Autodesk Inventor part; units mm, degrees
ref_plane "YZ Plane" through (0, 0, 0) normal (1, 0, 0) x (0, 1, 0)
ref_plane "XZ Plane" through (0, 0, 0) normal (0, 1, 0) x (-1, 0, 0)
ref_plane "XY Plane" through (0, 0, 0) normal (0, 0, 1) x (1, 0, 0)
sketch "Esboço1" plane through (0, 0, 0) normal (0, 1, 0) x (-1, 0, 0)
  line L0 (0, 0) -> (77, 0)
  line L1 (77, 0) -> (77, -140)
  line L2 (77, -140) -> (0, -140)
  line L3 (0, -140) -> (0, 0)
  circle A0 centre (67, -20) radius 2
  circle A1 centre (67, -120) radius 2
  circle A2 centre (26, -20) radius 2
  circle A3 centre (26, -120) radius 2
  dimension "d0" = 77
  dimension "d1" = 140
  dimension "d2" = 4
  dimension "d3" = 4
  dimension "d4" = 4
  dimension "d5" = 4
  dimension "d6" = 10
  dimension "d7" = 10
  dimension "d8" = 20
  dimension "d9" = 20
  dimension "d10" = 20
  dimension "d11" = 20
  dimension "d12" = 26
  dimension "d13" = 26
extrude "Extrusão1" add sketch "Esboço1" along normal blind 8
sketch "Esboço2" plane through (0, 8, 0) normal (0, 1, 0) x (1, 0, 0)
  circle A0 centre (-67, 20) radius 2
  circle A1 centre (-26, 20) radius 2
  circle A2 centre (-26, 120) radius 2
  circle A3 centre (-67, 120) radius 2
  circle A4 centre (-67, 20) radius 4
  circle A5 centre (-67, 120) radius 2
  circle A6 centre (-67, 120) radius 4.5
  circle A7 centre (-26, 120) radius 2
  circle A8 centre (-26, 120) radius 4.5
  circle A9 centre (-26, 20) radius 2
  circle A10 centre (-26, 20) radius 4.5
  point P0 (0, 0)
  dimension "d16" = 8
  dimension "d17" = 9
  dimension "d18" = 9
  dimension "d19" = 9
extrude "Extrusão2" cut sketch "Esboço2" against normal blind 3 contours A3 | A4 | A6 | A8 | A10
sketch "Esboço3" plane through (0, 8, 0) normal (0, 1, 0) x (1, 0, 0)
  point P0 (0, 0)
sketch "Esboço4" plane through (0, 8, 0) normal (0, 1, 0) x (1, 0, 0)
  circle A0 centre (-57, 30) radius 2
  circle A1 centre (-57, 110) radius 2
  circle A2 centre (-67, 20) radius 2
  circle A3 centre (-67, 120) radius 2
  circle A4 centre (-16, 30) radius 2
  circle A5 centre (-16, 110) radius 2
  circle A6 centre (-26, 20) radius 2
  circle A7 centre (-26, 120) radius 2
  point P0 (0, 0)
  dimension "d22" = 4
  dimension "d23" = 4
  dimension "d24" = 10
  dimension "d25" = 10
  dimension "d26" = 10
  dimension "d27" = 10
  dimension "d28" = 4
  dimension "d29" = 4
  dimension "d30" = 10
  dimension "d31" = 10
  dimension "d32" = 10
  dimension "d33" = 10
extrude "Extrusão3" cut sketch "Esboço4" against normal blind 12 contours A0 | A1 | A4 | A5
sketch "Esboço5" plane through (0, 0, 0) normal (0, -1, 0) x (1, 0, 0)
  circle A0 centre (-57, -110) radius 2
  circle A1 centre (-16, -110) radius 2
  circle A2 centre (-16, -30) radius 2
  circle A3 centre (-57, -30) radius 2
  line L0 (-53.525, -112.0063) -> (-57, -114.0126)
  line L1 (-57, -114.0126) -> (-60.475, -112.0063)
  line L2 (-60.475, -112.0063) -> (-60.475, -107.9937)
  line L3 (-60.475, -107.9937) -> (-57, -105.9874)
  line L4 (-57, -105.9874) -> (-53.525, -107.9937)
  line L5 (-53.525, -107.9937) -> (-53.525, -112.0063)
  line L6 (-53.525, -32.0063) -> (-57, -34.0126)
  line L7 (-57, -34.0126) -> (-60.475, -32.0063)
  line L8 (-60.475, -32.0063) -> (-60.475, -27.9937)
  line L9 (-60.475, -27.9937) -> (-57, -25.9874)
  line L10 (-57, -25.9874) -> (-53.525, -27.9937)
  line L11 (-53.525, -27.9937) -> (-53.525, -32.0063)
  line L12 (-16, -105.9874) -> (-12.525, -107.9937)
  line L13 (-12.525, -107.9937) -> (-12.525, -112.0063)
  line L14 (-12.525, -112.0063) -> (-16, -114.0126)
  line L15 (-16, -114.0126) -> (-19.475, -112.0063)
  line L16 (-19.475, -112.0063) -> (-19.475, -107.9937)
  line L17 (-19.475, -107.9937) -> (-16, -105.9874)
  circle A4 centre (-16, -30) radius 2
  line L18 (-12.525, -32.0063) -> (-16, -34.0126)
  line L19 (-16, -34.0126) -> (-19.475, -32.0063)
  line L20 (-19.475, -32.0063) -> (-19.475, -27.9937)
  line L21 (-19.475, -27.9937) -> (-16, -25.9874)
  line L22 (-16, -25.9874) -> (-12.525, -27.9937)
  line L23 (-12.525, -27.9937) -> (-12.525, -32.0063)
  line L24 (-77, -140) -> (-77, 0)
  line L25 (0, 0) -> (0, -140)
  dimension "d36" = 6.95
  dimension "d37" = 6.95
  dimension "d38" = 6.95
  dimension "d39" = 6.95
extrude "Extrusão4" cut sketch "Esboço5" against normal blind 5 contours A0 | L0 L1 L2 L3 L4 L5 | L6 L7 L8 L9 L10 L11 | L12 L13 L14 L15 L16 L17 | L18 L19 L20 L21 L22 L23
equation "\"d4\" = d3"
equation "\"d5\" = d3"
equation "\"d7\" = d6"
equation "\"d9\" = d8"
equation "\"d10\" = d9"
equation "\"d11\" = d8"
equation "\"d26\" = d25"
equation "\"d27\" = d26"
equation "\"d30\" = d24"
equation "\"d33\" = d32"
equation "\"d36\" = d39"
equation "\"d37\" = d39"
equation "\"d38\" = d39"
properties part number "suporte-fonte"
Read the model definition and answer for the solid it produces. Units are mm, in the model's axes. A direction names the side the tool comes from. Give positions to 0.01 mm unless a question says otherwise; leave off trailing zeros. Loops run counter-clockwise (first coordinate to the right, second up) from the corner with the lowest first, then second, coordinate; pieces in that order, holes last. Notation, with made-up numbers: (47.25, 80) - (64.25, 80) arc R26 ccw to (64.25, 94) - close; hole circle Ø4 at (-7, 76.25). An arc over 180 degrees is marked (long way). Answer as CSV lines item,"result". Start each with the question number.
1) Each of these flat-tipped pins is pushed along its axis until it touches: pin 1 Ø4.5 at (y, z) = (3.5, -111) entering from +X; pin 2 Ø4.5 at (x, z) = (-25.5, -18.5) entering from +Y; pin 3 Ø5 at (x, z) = (-57, -110) entering from -Y. Where does it stop, or does it pass through?
2) Find section C-C (y = 2.25). State how many separate pieces and enclosed holes the cut face has, then the cut area to 3 significant figures.
3) Which of the six approach directions +Z, -Z, +X, -X, +Y, -Y give full straight-line access (tool end or side, diameter ignored) to faces 3 (the face through (-18, 5, -32)), 4 (the face through (-25, 5, -18)), 5 (the face through (-16, 7, -112))?
4) Find section B-B (x = -26). Write down the section's boundary in (y, z), then the cut area to 3 significant figures.
5) Find section A-A (z = -120). Write down the section's boundary in (x, y), then the cut area to 3 significant figures.
6) Straight lines are drawn through the part: L1, parallel to X at y = 6.05, z = -20; L2, parallel to X at y = 7.05, z = -110; L3, parallel to Z at x = -26, y = 2.65. For each, find the intervals that lie inside material, in ascending order. Write a range as from..to.
7) Determine the mould class of faces 1 (the face through (-38, 4, 0)), 2 (the face through (-58.762, 2.465, -27.005)) for opening direction Z: released by +Z, released by -Z, zero draft, split by the parting line, or undercut.
Findings below:
1,pin 1,"x = 0"
1,pin 2,"y = 5"
1,pin 3,"y = 5"
2,separate pieces,"1"
2,enclosed holes,"8"
2,area,"10,600 mm^2"
3,face 3,"-Y"
3,face 4,"+Y"
3,face 5,"+Y, -Y"
4,outline,"(0, -140) - (8, -140) - (8, -124.5) - (5, -124.5) - (5, -122) - (0, -122) - close; (0, -118) - (5, -118) - (5, -115.5) - (8, -115.5) - (8, -24.5) - (5, -24.5) - (5, -22) - (0, -22) - close; (0, -18) - (5, -18) - (5, -15.5) - (8, -15.5) - (8, 0) - (0, 0) - close"
4,area,"1,030 mm^2"
5,outline,"(-77, 0) - (-69, 0) - (-69, 5) - (-71.5, 5) - (-71.5, 8) - (-77, 8) - close; (-65, 0) - (-28, 0) - (-28, 5) - (-30.5, 5) - (-30.5, 8) - (-62.5, 8) - (-62.5, 5) - (-65, 5) - close; (-24, 0) - (0, 0) - (0, 8) - (-21.5, 8) - (-21.5, 5) - (-24, 5) - close"
5,area,"522 mm^2"
6,L1,"-77..-71, -63..-30.5, -21.5..0"
6,L2,"-77..-59, -55..-18, -14..0"
6,L3,"-140..-122, -118..-22, -18..0"
7,face 1,"released by +Z"
7,face 2,"undercut"
